Autodesk Inventor part; units mm, degrees
ref_plane "Work Plane1" through (0.8, 0, 0) normal (1, 0, 0) x (0, 0, -1)
ref_plane "YZ Plane" through (0, 0, 0) normal (1, 0, 0) x (0, 1, 0)
ref_plane "XZ Plane" through (0, 0, 0) normal (0, 1, 0) x (-1, 0, 0)
sketch "Sketch1" plane through (0, 0, 0) normal (0, 1, 0) x (-1, 0, 0)
  line L0 (0, 0) -> (34.5, 0)
  line L1 (34.5, 0) -> (34.5, -17.6)
  line L2 (34.5, -17.6) -> (0, -17.6)
  line L3 (0, -17.6) -> (0, 0)
  dimension "d0" = 17.6
  dimension "d1" = 34.5
extrude "Extrusion1" add sketch "Sketch1" along normal blind 1.05
ref_plane "Work Plane1" through (0.8, 0, 0) normal (1, 0, 0) x (0, 0, -1)
sketch "Sketch2" plane through (0.8, 0, 0) normal (1, 0, 0) x (0, 0, -1)
  line L0 (0, 0) -> (17.6, 0)
  line L1 (17.6, 0) -> (17.6, 1.05)
  line L2 (0, 1.05) -> (17.6, 1.05)
  line L3 (0, 0) -> (0, 1.05)
  line L4 (17.6, 0) -> (0, 0) construction
  line L5 (8.8, 0) -> (8.8, 1.05) construction
  line L6 (17.6, 1.05) -> (0, 1.05) construction
  line L7 (5.34, 4.22) -> (12.26, 4.22)
  line L8 (13.3, 3.18) -> (13.3, 2.09)
  line L9 (12.26, 1.05) -> (5.34, 1.05)
  line L10 (4.3, 2.09) -> (4.3, 3.18)
  line L11 (0, 1.05) -> (17.6, 1.05)
  arc A0 (5.34, 4.22) -> (4.3, 3.18) centre (5.34, 3.18) ccw
  arc A1 (4.3, 2.09) -> (5.34, 1.05) centre (5.34, 2.09) ccw
  arc A2 (13.3, 3.18) -> (12.26, 4.22) centre (12.26, 3.18) ccw
  arc A3 (12.26, 1.05) -> (13.3, 2.09) centre (12.26, 2.09) ccw
  point P0 (4.3, 4.22)
  point P1 (13.3, 4.22)
  point P2 (4.3, 1.05)
  point P3 (5.34, 1.05)
  point P4 (12.26, 1.05)
  dimension "d5" = 9
  dimension "d6" = 3.17
  dimension "d7" = 1.04
extrude "Extrusion2" add sketch "Sketch2" against normal blind 7.35 contours A1 L10 A0 L7 A2 L8 A3 L2
equation "\"d2\" = pcbThickness"
equation "\"pcbThickness\" = 1.05"
equation "\"usbcEdgeOffset\" = 0.8"
equation "\"d4\" = usbcEdgeOffset"
properties part number "MCU_TinyPICO"
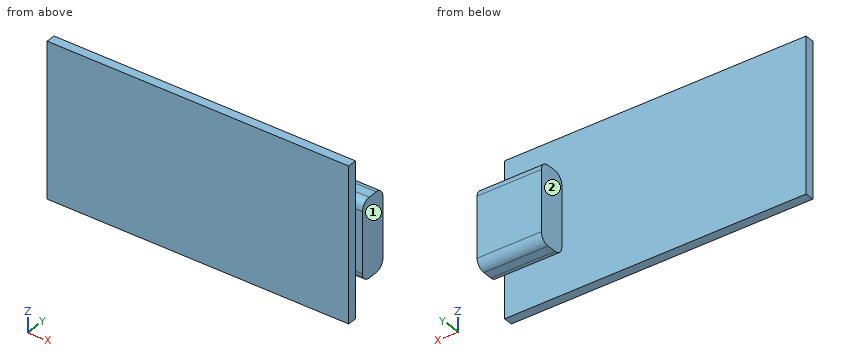
Could you check a few things on this model? Use its own coordinates, in mm. Face numbers are marked on the shaded views. A direction names the side the tool comes from. Give positions to 0.01 mm unless a question says otherwise; leave off trailing zeros. Loops run counter-clockwise (first coordinate to the right, second up) from the corner with the lowest first, then second, coordinate; pieces in that order, holes last. Notation, with made-up numbers: (74, 55.5) -> (95, 55.5) arc R15 ccw to (95, 76.5) -> close; hole circle Ø4 at (64, 37.25). An arc over 180 degrees is marked (long way). Put each result on its own line as item: value.
(1) For the marked faces 1 and 2, which set-ups out of +Z, -Z, +X, -X, +Y, -Y let a thin tool reach every point of the face, with its end or its side?
Computed:
face 1: +Z, -Z, +X, +Y, -Y
face 2: +Z, -Z, -X, +Y
(2) Imagine slicing it at B-B on z = -7.5. Write out the boundary of the cut face in (x, y), plus the area to 3 significant figures.
Computed:
outline: (-34.5, 0) -> (0, 0) -> (0, 1.05) -> (0.8, 1.05) -> (0.8, 4.22) -> (-6.55, 4.22) -> (-6.55, 1.05) -> (-34.5, 1.05) -> close
area: 59.5 mm^2
(3) Imagine slicing it at C-C on y = 0.45. Write out the boundary of the cut face in (x, z).
Computed:
outline: (-34.5, -17.6) -> (0, -17.6) -> (0, 0) -> (-34.5, 0) -> close
(4) Please list where these lines run through material, in increasing order: probe 1 along Y at (x, z) = (-18, -5); probe 2 along X at (y, z) = (0.7, -6.5); probe 3 along X at (y, z) = (1.85, -12.25). Write a range as [from, to].
Computed:
probe 1: [0, 1.05]
probe 2: [-34.5, 0]
probe 3: [-6.55, 0.8]
(5) Imagine slicing it at D-D on x = -31. Write out the boundary of the cut face in (y, z).
Computed:
outline: (0, -17.6) -> (1.05, -17.6) -> (1.05, 0) -> (0, 0) -> close
(6) Imagine slicing it at A-A on z = -4.75. Write out the boundary of the cut face in (x, y).
Computed:
outline: (-34.5, 0) -> (0, 0) -> (0, 1.05) -> (-34.5, 1.05) -> close; (-6.55, 1.23) -> (0.8, 1.23) -> (0.8, 4.04) -> (-6.55, 4.04) -> close
(7) I'm going to push flat-ended pins straight in: pin 1 Ø0.8 at (y, z) = (0.5, -10.5) entering from +X; pin 2 Ø2 at (x, z) = (-7, -14.5) entering from +Y; pin 3 Ø2.5 at (y, z) = (2.5, -10) entering from -X; pin 4 Ø2 at (y, z) = (3, -3) entering from +X. Where does each tip first touch, or does it pass through?
Computed:
pin 1: x = 0
pin 2: y = 1.05
pin 3: x = -6.55
pin 4: through
